Input: part model. Units: mm. Frame: model coordinates. A direction names the side the tool comes from. Round coordinates to 2 decimals unless told otherwise and drop trailing zeros. Order: outer loops, then holes, each group sorted by start corner. A loop starts at its lowest first (then second) coordinate and runs counter-clockwise, first axis right, second up.
Item 1: Cut plane C-C on y = 1.75. Output: boundary loops of the cut face in (x, z).
Item 2: Cut plane D-D on x = 27.5. Output: boundary loops of the cut face in (y, z), then the cut area to 3 significant figures.
Item 3: First-contact query: pin 1 (2 mm diameter, centred on y = 3, z = -18.5, fed in from +X); pin 2 (12 mm diameter, centred on x = 45.5, z = 31.5, fed in from -Y); pin 3 (4.5 mm diameter, centred on y = 1, z = 32.5, fed in from -X); pin 4 (3 mm diameter, centred on x = 24.5, y = 4, fed in from -Z). Flat tips, straight axial feed; report the tip coordinate or a pass-through.
Item 4: Cut plane A-A on x = -46.5. Output: boundary loops of the cut face in (y, z).
Item 5: Line query: L1, parallel to Z at x = 23, y = 1.75; L2, parallel to X at y = 0.75, z = 23.5; L3, parallel to X at y = 7.25, z = -20.5. Output: solid intervals per line, ascending.
Item 6: Mould query, pull axis X, two halves, no side actions, for faces 1 (the flat face through (21, 2, 16.948)), 2 (the flat face through (-55.289, 3, -3)), 3 (the flat face through (0, 3, -47.652)). Classes: released by +X, released by -X, zero draft, split by the parting line, or undercut.
Item 7: Reachability of faces 4 (the flat face through (-4, 0, 8)), 5 (the flat face through (0, 3, 43.548)), 6 (the flat face through (-39, 2, 16.948)), 7 (the flat face through (-1, 8, -52.052)), 8 (the flat face through (0, 5, 4.948)) from +Z, -Z, +X, -X, +Y, -Y: full face, straight path, thin tool, end or side. Return the list, or none.
Item 8: Cut plane B-B on z = -13.5. Output: boundary loops of the cut face in (x, y).
```python
from build123d import *

# Parameters (mm, degrees)
SKETCH1_W           = 120
SKETCH1_H           = 100
BOSS_EXTRUDE1_DEPTH = 10
SKETCH2_W           = 98.5
SKETCH2_H           = 42
CUT_EXTRUDE1_DEPTH  = 10
SKETCH3_W           = 120
SKETCH3_H           = 100
SKETCH3_W_2         = 111.2
SKETCH3_H_2         = 91.2
CUT_EXTRUDE3_DEPTH  = 7
SKETCH4_W           = 18
SKETCH4_H           = 25
CUT_EXTRUDE4_DEPTH  = 4
SKETCH5_W           = 3
SKETCH5_H           = 25
CUT_EXTRUDE6_DEPTH  = 2.5
SKETCH6_R           = 4
CUT_EXTRUDE12_DEPTH = 80.892767694


with BuildPart() as part:
    # Sketch1 → Boss-Extrude1 (new body)
    with BuildSketch(Plane(origin=(0, 0, 0), x_dir=(1, 0, 0), z_dir=(0, 1, 0))):
        with Locations((0.311320755, 2.051886792)):
            Rectangle(SKETCH1_W, SKETCH1_H)
    extrude(amount=BOSS_EXTRUDE1_DEPTH)

    # Sketch2 → Cut-Extrude1 (cut)
    with BuildSketch(Plane(origin=(0, 10, 0), x_dir=(1, 0, 0), z_dir=(0, 1, 0))):
        with Locations((0.811320755, 16.051886792)):
            Rectangle(SKETCH2_W, SKETCH2_H)
    extrude(amount=-CUT_EXTRUDE1_DEPTH, mode=Mode.SUBTRACT)

    # Sketch3 → Cut-Extrude3 (cut)
    with BuildSketch(Plane.XZ):
        with Locations((0.311320755, -2.051886792)):
            Rectangle(SKETCH3_W, SKETCH3_H)
        with Locations((0.311320755, -2.051886792)):
            Rectangle(SKETCH3_W_2, SKETCH3_H_2, mode=Mode.SUBTRACT)
    extrude(amount=-CUT_EXTRUDE3_DEPTH, mode=Mode.SUBTRACT)

    # Sketch4 → Cut-Extrude4 (cut)
    with BuildSketch(Plane.XZ):
        with Locations((-39.17934754, 29.448113208)):
            Rectangle(SKETCH4_W, SKETCH4_H)
        with Locations((-19.133803456, 29.448113208)):
            Rectangle(SKETCH4_W, SKETCH4_H)
        with Locations((0.911740628, 29.448113208)):
            Rectangle(SKETCH4_W, SKETCH4_H)
        with Locations((20.957284712, 29.448113208)):
            Rectangle(SKETCH4_W, SKETCH4_H)
        with Locations((41.002828796, 29.448113208)):
            Rectangle(SKETCH4_W, SKETCH4_H)
    extrude(amount=-CUT_EXTRUDE4_DEPTH, mode=Mode.SUBTRACT)

    # Sketch5 → Cut-Extrude6 (cut)
    with BuildSketch(Plane.XZ.offset(-4)):
        with Locations((33.502828796, 29.448113208)):
            Rectangle(SKETCH5_W, SKETCH5_H)
        with Locations((13.457284712, 29.448113208)):
            Rectangle(SKETCH5_W, SKETCH5_H)
        with Locations((-6.588259372, 29.448113208)):
            Rectangle(SKETCH5_W, SKETCH5_H)
        with Locations((-26.633803456, 29.448113208)):
            Rectangle(SKETCH5_W, SKETCH5_H)
        with Locations((-46.67934754, 29.448113208)):
            Rectangle(SKETCH5_W, SKETCH5_H)
    extrude(amount=-CUT_EXTRUDE6_DEPTH, mode=Mode.SUBTRACT)

    # Sketch6 → Cut-Extrude12 (cut, through all)
    with BuildSketch(Plane.XZ.offset(-4)):
        with Locations(Location((41.502828796, 26.198113208, 0), (0, 0, 270))):
            Circle(SKETCH6_R)
        with Locations(Location((21.457284712, 26.198113208, 0), (0, 0, 270))):
            Circle(SKETCH6_R)
        with Locations(Location((1.411740628, 26.198113208, 0), (0, 0, 270))):
            Circle(SKETCH6_R)
        with Locations(Location((-18.633803456, 26.198113208, 0), (0, 0, 270))):
            Circle(SKETCH6_R)
        with Locations(Location((-38.67934754, 26.198113208, 0), (0, 0, 270))):
            Circle(SKETCH6_R)
    extrude(amount=-CUT_EXTRUDE12_DEPTH, mode=Mode.SUBTRACT)


solid = part.part
```
From the geometry:
1. outline: (-55.29, -47.65) - (55.91, -47.65) - (55.91, 43.55) - (-55.29, 43.55) - close; hole (-48.44, -37.05) - (50.06, -37.05) - (50.06, 4.95) - (-48.44, 4.95) - close; hole (-48.18, 16.95) - (-30.18, 16.95) - (-30.18, 41.95) - (-48.18, 41.95) - close; hole (-28.13, 16.95) - (-10.13, 16.95) - (-10.13, 41.95) - (-28.13, 41.95) - close; hole (-8.09, 16.95) - (9.91, 16.95) - (9.91, 41.95) - (-8.09, 41.95) - close; hole (11.96, 16.95) - (29.96, 16.95) - (29.96, 41.95) - (11.96, 41.95) - close; hole (32, 16.95) - (50, 16.95) - (50, 41.95) - (32, 41.95) - close
2. outline: (0, -47.65) - (7, -47.65) - (7, -52.05) - (10, -52.05) - (10, -37.05) - (0, -37.05) - close; (0, 4.95) - (10, 4.95) - (10, 47.95) - (7, 47.95) - (7, 43.55) - (0, 43.55) - (0, 41.95) - (4, 41.95) - (4, 16.95) - (0, 16.95) - close
2. area: 418 mm2
3. pin 1: stops at x = 55.91
3. pin 2: stops at y = 0
3. pin 3: stops at x = -55.29
3. pin 4: stops at z = -47.65
4. outline: (0, -47.65) - (7, -47.65) - (7, -52.05) - (10, -52.05) - (10, -37.05) - (0, -37.05) - close; (0, 4.95) - (10, 4.95) - (10, 47.95) - (7, 47.95) - (7, 43.55) - (0, 43.55) - (0, 41.95) - (6.5, 41.95) - (6.5, 16.95) - (0, 16.95) - close
5. L1: z = -47.65 to -37.05, 4.95 to 16.95, 41.95 to 43.55
5. L2: x = -55.29 to -48.18, -30.18 to -28.13, -10.13 to -8.09, 9.91 to 11.96, 29.96 to 32, 50 to 55.91
5. L3: x = -59.69 to -48.44, 50.06 to 60.31
6. face 1: undercut
6. face 2: released by -X
6. face 3: zero draft
7. face 4: +Z, -Z, +X, -X, -Y
7. face 5: +Z, +X, -X, -Y
7. face 6: -Y
7. face 7: -Z, +X, -X, +Y, -Y
7. face 8: +Y, -Y
8. outline: (-59.69, 7) - (-55.29, 7) - (-55.29, 0) - (-48.44, 0) - (-48.44, 10) - (-59.69, 10) - close; (50.06, 0) - (55.91, 0) - (55.91, 7) - (60.31, 7) - (60.31, 10) - (50.06, 10) - close
